Check sheet for the modelled part. Datum: model origin and axes. Units: mm. Face numbers are marked on the shaded views. Round coordinates to 2 decimals unless told otherwise and drop trailing zeros. Order: outer loops, then holes, each group sorted by start corner. A loop starts at its lowest first (then second) coordinate and runs counter-clockwise, first axis right, second up.
```python
from build123d import *

# Parameters (mm, degrees)
SKETCH1_R           = 23
BOSS_EXTRUDE1_DEPTH = 5
SKETCH2_R           = 3.125
CUT_EXTRUDE1_DEPTH  = 6
SKETCH4_W           = 22.031580043
SKETCH4_H           = 3
CUT_EXTRUDE2_DEPTH  = 6


with BuildPart() as part:
    # Sketch1 → Boss-Extrude1 (new body)
    with BuildSketch(Plane.XY):
        Circle(SKETCH1_R)
    extrude(amount=BOSS_EXTRUDE1_DEPTH)

    # Sketch2 → Cut-Extrude1 (cut, through all)
    with BuildSketch(Plane(origin=(0, 0, 0), x_dir=(-1, 0, 0), z_dir=(0, 0, -1))):
        Circle(SKETCH2_R)
    extrude(amount=-CUT_EXTRUDE1_DEPTH, mode=Mode.SUBTRACT)

    # Sketch4 → Cut-Extrude2 (cut, through all)
    with BuildSketch(Plane(origin=(0, 0, 0), x_dir=(-1, 0, 0), z_dir=(0, 0, -1))):
        with Locations((13.757254046, 0)):
            Rectangle(SKETCH4_W, SKETCH4_H)
    extrude(amount=-CUT_EXTRUDE2_DEPTH, mode=Mode.SUBTRACT)


solid = part.part
```
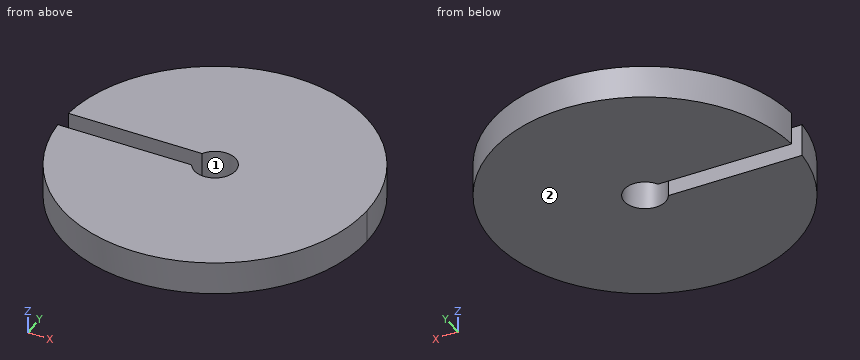
Item 1: Go/stop test with flat-tipped pins: P1, Ø2, axis at x = 4, z = 2.5, coming from the -Y side; P2, Ø1.5, axis at x = -17.5, z = 2, coming from the +Y side; P3, Ø2, axis at y = 15, z = 4, coming from the +X side. Record where each tip stops, or that it passes through.
Answer:
P1: stops at y = -22.8
P2: stops at y = 15.76
P3: stops at x = 18.25
Item 2: Sectioned sample at B-B (z = 3.9). Record the cut outline in (x, y) (3 decimals).
Answer:
outline: (-22.951, -1.5) arc R23 ccw (long way) to (-22.951, 1.5) - (-2.741, 1.5) arc R3.125 cw (long way) to (-2.741, -1.5) - close
Item 3: Sectioned sample at C-C (y = -17). Record the cut outline in (x, z), and give its area (3 significant figures).
Answer:
outline: (-15.49, 0) - (15.49, 0) - (15.49, 5) - (-15.49, 5) - close
area: 155 mm2
Item 4: Scan lines: line 1 along Y through (x, z) = (0, 1.8) (3 decimals); line 2 along X through (y, z) = (0, 3.8) (3 decimals); line 3 along Y through (x, z) = (-14.5, 4.1). Record each from-to range of solid material in increasing order.
Answer:
line 1: y = -23 to -3.125, 3.125 to 23
line 2: x = 3.125 to 23
line 3: y = -17.85 to -1.5, 1.5 to 17.85
Item 5: Sectioned sample at D-D (x = -5). Record the cut outline in (y, z).
Answer:
outline: (-22.45, 0) - (-1.5, 0) - (-1.5, 5) - (-22.45, 5) - close; (1.5, 0) - (22.45, 0) - (22.45, 5) - (1.5, 5) - close
Item 6: Sectioned sample at A-A (x = 0). Record the cut outline in (y, z) (3 decimals).
Answer:
outline: (-23, 0) - (-3.125, 0) - (-3.125, 5) - (-23, 5) - close; (3.125, 0) - (23, 0) - (23, 5) - (3.125, 5) - close
Item 7: Release check for a two-part mould opening along X. For the marked faces 1 and 2 record: released by +X, released by -X, zero draft, split by the parting line, or undercut.
Answer:
face 1: undercut
face 2: zero draft
